Input: part model. Units: mm. Frame: model coordinates. Coordinates: 2 decimals unless noted, no trailing zeros. Loops run counter-clockwise (first coordinate to the right, second up) from the corner with the lowest first, then second, coordinate; pieces in that order, holes last.
```python
from build123d import *

# Parameters (mm, degrees)
SKETCH2_R               = 24.97201
SKETCH2_R_2             = 21.79701
EXTRUDE_THIN1_DEPTH     = 1054.1
SKETCH3_R               = 3.175
CUT_EXTRUDE2_DEPTH      = 25.97201
CUT_EXTRUDE2_DEPTH_BACK = 25.97201


with BuildPart() as part:
    # Sketch2 → Extrude-Thin1 (new body)
    with BuildSketch(Plane(origin=(0, 0, 0), x_dir=(1, 0, 0), z_dir=(0, 1, 0))):
        Circle(SKETCH2_R)
        Circle(SKETCH2_R_2, mode=Mode.SUBTRACT)
    extrude(amount=EXTRUDE_THIN1_DEPTH)

    # Sketch3 → Cut-Extrude2 (cut, two sides)
    with BuildSketch(Plane.XY) as cut_extrude2_sk:
        with Locations((0, 12.7)):
            Circle(SKETCH3_R)
        with Locations((0, 1038.225)):
            Circle(SKETCH3_R)
    extrude(amount=CUT_EXTRUDE2_DEPTH, mode=Mode.SUBTRACT)
    extrude(cut_extrude2_sk.sketch, amount=-CUT_EXTRUDE2_DEPTH_BACK, mode=Mode.SUBTRACT)


solid = part.part
```
Item 1: Contact query for flat-ended pins moving along their axis: P1, Ø5, axis at y = 871, z = 18.5, coming from the +X side; P2, Ø6, axis at y = 331, z = -9, coming from the -X side; P3, Ø8, axis at x = 12.5, y = 158, coming from the -Z side; P4, Ø5, axis at x = 0, y = 12.7, coming from the +Z side. Output: stop coordinate, or through.
Result:
P1: stops at x = 19.17
P2: stops at x = -24.24
P3: stops at z = -23.48
P4: passes through
Item 2: Section query B-B (y = 582). Output: boundary loops of the cut face in (x, z).
Result:
outline: circle Ø49.94 at (0, 0); hole circle Ø43.59 at (0, 0)
Item 3: Section query A-A (z = 0). Output: boundary loops of the cut face in (x, y).
Result:
outline: (-24.97, 0) - (-21.8, 0) - (-21.8, 1054.1) - (-24.97, 1054.1) - close; (21.8, 0) - (24.97, 0) - (24.97, 1054.1) - (21.8, 1054.1) - close
Item 4: Line query: L1, parallel to Y at x = 0, z = -22.5 (3 decimals); L2, parallel to Z at x = 0.5, y = 740.5. Output: solid intervals per line, ascending.
Result:
L1: y = 0 to 9.525, 15.875 to 1035.05, 1041.4 to 1054.1
L2: z = -24.97 to -21.79, 21.79 to 24.97
